Part model, mm, in its own coordinate system. A direction names the side the tool comes from. Give positions to 0.01 mm unless a question says otherwise; leave off trailing zeros. Write each loop counter-clockwise with the first axis right and the second up, starting at its lowest first coordinate (ties: lowest second). Pieces come first, ordered by that corner, then holes. Notation, with made-up numbers: M 15.5,17 L 24.5,17 A13 cw 24.5,40 Z; hole C 51.25,2.25 d5. An arc over 180 degrees is marked long. Use a Markdown table: item, result. Add a question column.
Autodesk Fusion 360 part; units mm, degrees
sketch "Sketch1" plane through (0, 0, 0) normal (0, 1, 0) x (1, 0, 0)
  line L0 (-102.9234, -55.5196) -> (-38.7234, -55.5196)
  line L1 (-38.7234, -55.5196) -> (-38.7234, -11.4886)
  line L2 (-38.7234, -11.4886) -> (-102.9234, -11.4886)
  line L3 (-102.9234, -11.4886) -> (-102.9234, -55.5196)
  line L4 (-112.4234, -65.0196) -> (-29.2234, -65.0196)
  line L5 (-29.2234, -65.0196) -> (-29.2234, -1.9886)
  line L6 (-29.2234, -1.9886) -> (-112.4234, -1.9886)
  line L7 (-112.4234, -1.9886) -> (-112.4234, -65.0196)
  circle A0 centre (-107.4234, -60.0196) radius 1.7
  circle A1 centre (-34.2234, -60.0196) radius 1.7
  circle A2 centre (-107.4234, -6.9886) radius 1.7
  circle A3 centre (-34.2234, -6.9886) radius 1.7
  circle A4 centre (-107.4234, -60.0196) radius 3
  circle A5 centre (-107.4234, -6.9886) radius 3
  circle A6 centre (-34.2234, -6.9886) radius 3
  circle A7 centre (-34.2234, -60.0196) radius 3
  dimension "d1" = 64.2
  dimension "d2" = 44.031
  dimension "d3" = 83.2
  dimension "d4" = 63.031
  dimension "d5" = 9.5
  dimension "d6" = 9.5
  dimension "d7" = 3.4
  dimension "d8" = 3.4
  dimension "d9" = 3.4
  dimension "d10" = 3.4
  dimension "d11" = 5
  dimension "d12" = 5
  dimension "d13" = 5
  dimension "d14" = 5
  dimension "d15" = 5
  dimension "d16" = 5
  dimension "d17" = 5
  dimension "d18" = 5
  dimension "d19" = 6
  dimension "d20" = 6
  dimension "d21" = 6
  dimension "d22" = 6
extrude "Extrude1" add sketch "Sketch1" along normal blind 9.9 from surface at 3.1 contours A4 | A5 | A6 | A7 makes body 1 at (-37.2197, 9.7, 60.1692) makes body 2 at (-31.2271, 9.7, 7.1382) makes body 3 at (-109.5181, 9.7, 62.1672) makes body 4 at (-104.4271, 9.7, 7.1382)
extrude "Extrude2" add sketch "Sketch1" along normal blind 13 contours L4 L5 L6 L7 bodies 1 2 3 4
extrude "Extrude3" add sketch "Sketch1" along normal blind 3 contours L0 L1 L2 L3 bodies 1
sketch "Sketch2" plane through (0, 13, 0) normal (0, 1, 0) x (-1, 0, 0)
  circle A0 centre (34.2234, 60.0196) radius 1.7
  circle A1 centre (107.4234, 6.9886) radius 1.7
  line L0 (102.9234, 55.5196) -> (102.9234, 11.4886)
  line L1 (102.9234, 11.4886) -> (38.7234, 11.4886)
  line L2 (38.7234, 11.4886) -> (38.7234, 55.5196)
  line L3 (38.7234, 55.5196) -> (102.9234, 55.5196)
  line L4 (112.4234, 1.9886) -> (112.4234, 65.0196)
  line L5 (112.4234, 65.0196) -> (29.2234, 65.0196)
  line L6 (29.2234, 65.0196) -> (29.2234, 1.9886)
  line L7 (29.2234, 1.9886) -> (112.4234, 1.9886)
  circle A2 centre (34.2234, 6.9886) radius 1.7
  circle A3 centre (107.4234, 60.0196) radius 1.7
  line L8 (29.2234, 23.7386) -> (38.7234, 23.7386)
  line L9 (38.7234, 23.7386) -> (38.7234, 42.2386)
  line L10 (38.7234, 42.2386) -> (29.2234, 42.2386)
  line L11 (29.2234, 42.2386) -> (29.2234, 23.7386)
  line L12 (29.2234, 1.9886) -> (112.4234, 1.9886)
  dimension "d30" = 18.5
  dimension "d31" = 21.75
extrude "Extrude4" cut sketch "Sketch2" against normal blind 7.5 contours L2 L6 L8 L9 L10 L11 bodies 1
fillet "Fillet1" radius 5 1 edges at (-112.4234, 6.5, 65.0196) on bodies 1
fillet "Fillet2" radius 5 1 edges at (-112.4234, 6.5, 1.9886) on bodies 1
fillet "Fillet3" radius 5 1 edges at (-29.2234, 6.5, 65.0196) on bodies 1
1. Mould opens along X. For faces 5 (the flat face through (-102.923, 8, 33)), 6 (the flat face through (-68, 6, 1.989)), 7 (the cylindrical face through (-110.92, 6.591, 3.414)) say: released by +X, released by -X, zero draft, split by the parting line, or undercut.
2. Cut at D-D (x = -50). Write the cut outline in (y, z), then the cut area to 3 significant figures.
3. Cut at A-A (y = 4.25). Write the cut outline in (x, z).
4. Drill centre lines: probe 1 along Z at (x, y) = (-63, 5.5); probe 2 along X at (y, z) = (5, 31); probe 3 along X at (y, z) = (12.25, 6.5). Where is each one in solid material? Low to high. Write a range as [from, to].
5. Flat gauge pins, fed straight in: pin 1 (6.5 mm diameter, centred on x = -107.5, z = 59, fed in from -Y); pin 2 (3 mm diameter, centred on x = -33, z = 33.5, fed in from +Y); pin 3 (5.5 mm diameter, centred on x = -107.42, z = 6.99, fed in from -Y); pin 4 (2 mm diameter, centred on x = -107.42, z = 6.99, fed in from +Y). Where does each tip first touch, or does it go through?
6. Tool access for faces 1 (the flat face through (-71, 8, 55.52)), 2 (the cylindrical face through (-32.61, 1.53, 62.55)), 3 (the cylindrical face through (-32.602, 7.981, 7.499)), 4 (the flat face through (-34, 5.5, 33)): list every direction of +Z, -Z, +X, -X, +Y, -Y with a clear straight run to the whole face (end or side of a thin tool).
7. Cut at B-B (z = 49). Write the cut outline in (x, y), then the cut area to 3 significant figures.
8. Cut at C-C (y = 11.75). Write the cut outline in (x, z).
A:
| question | item | result |
|---|---|---|
| 1 | face 5 | undercut |
| 1 | face 6 | zero draft |
| 1 | face 7 | released by -X |
| 2 | outline | M 0,1.99 L 13,1.99 L 13,11.49 L 3,11.49 L 3,55.52 L 13,55.52 L 13,65.02 L 0,65.02 Z |
| 2 | area | 379 mm² |
| 3 | outline | M -112.42,6.99 A5 ccw -107.42,1.99 L -29.22,1.99 L -29.22,60.02 A5 ccw -34.22,65.02 L -107.42,65.02 A5 ccw -112.42,60.02 Z; hole C -107.42,6.99 d3.4; hole C -107.42,60.02 d3.4; hole M -102.92,11.49 L -38.72,11.49 L -38.72,55.52 L -102.92,55.52 Z; hole C -34.22,6.99 d3.4; hole C -34.22,60.02 d3.4 |
| 4 | probe 1 | z = [1.99, 11.49], [55.52, 65.02] |
| 4 | probe 2 | x = [-112.42, -102.92], [-38.72, -29.22] |
| 4 | probe 3 | x = [-112.4, -109.05], [-105.8, -35.85], [-32.6, -29.22] |
| 5 | pin 1 | stops at y = 0 |
| 5 | pin 2 | stops at y = 5.5 |
| 5 | pin 3 | stops at y = 3.1 |
| 5 | pin 4 | passes through |
| 6 | face 1 | +Y |
| 6 | face 2 | -Y |
| 6 | face 3 | +Y, -Y |
| 6 | face 4 | +X, +Y |
| 7 | outline | M -112.42,0 L -29.22,0 L -29.22,13 L -38.72,13 L -38.72,3 L -102.92,3 L -102.92,13 L -112.42,13 Z |
| 7 | area | 440 mm² |
| 8 | outline | M -112.42,6.99 A5 ccw -107.42,1.99 L -29.22,1.99 L -29.22,23.74 L -38.72,23.74 L -38.72,11.49 L -102.92,11.49 L -102.92,55.52 L -38.72,55.52 L -38.72,42.24 L -29.22,42.24 L -29.22,60.02 A5 ccw -34.22,65.02 L -107.42,65.02 A5 ccw -112.42,60.02 Z; hole C -107.42,6.99 d3.4; hole C -107.42,60.02 d3.4; hole C -34.22,6.99 d3.4; hole C -34.22,60.02 d3.4 |
